Could you check a few things on this model? Use its own coordinates, in mm. Face numbers are marked on the shaded views. Give positions to 0.01 mm unless a question says otherwise; leave off trailing zeros. Loops run counter-clockwise (first coordinate to the right, second up) from the corner with the lowest first, then second, coordinate; pieces in that order, holes last. Notation, with made-up numbers: M -34.75,75.5 L -17.75,75.5 A5 ccw -17.75,82.5 Z; hole C -40,-17.75 d5. An arc over 180 degrees is marked long. Answer in a Markdown table with one row per item. Add a question column.
1. Thinking about a two-plate mould opening in Y: for the marked faces 1 and 2, which applies, released by +Y, released by -Y, zero draft, split by the parting line, or undercut?
2. If we section it at B-B on x = -14: List the corners of the cut face in (y, z) for me, then the cut area to 3 significant figures.
3. If we section it at A-A on z = 4.25: List the corners of the cut face in (x, y) for me (3 decimals).
4. I need wall thicknesses on line 1 along Y through (x, z) = (-20.5, 5.75); line 2 along Y through (x, z) = (-5.5, 5.5); line 3 along X through (y, z) = (6, 1). Which ranges of each line are inside material? Lowest first, please. Write a range as from..to.
5. I'm going to push flat-ended pins straight in: pin 1 Ø1 at (y, z) = (-6.5, 0.5) entering from -X; pin 2 Ø2 at (x, z) = (-8, 3.5) entering from +Y; pin 3 Ø1.5 at (y, z) = (30.5, 5.5) entering from -X. Where does each tip first touch, or does it pass through?
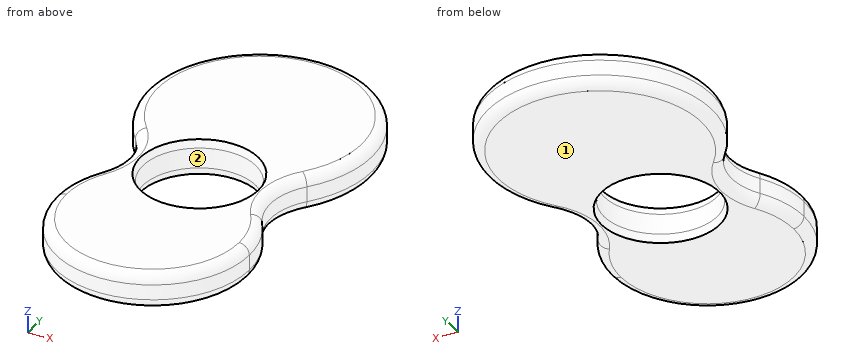
```python
from build123d import *

# Parameters (mm, degrees)
F0_R     = 11.1
F1_DEPTH = 7
F2_SIZE2 = 0.5
F2_SIZE  = 1.5
F3_R     = 2


with BuildPart() as f1:
    # F0 (on Top) → F1 (new body)
    with BuildSketch(Plane.XY):
        with BuildLine():
            ThreePointArc((-30.871365, 7.905008), (-28.023647, 0.762863), (-29.966515, -6.676558))
            ThreePointArc((-29.966515, -6.676558), (-32.225858, -11.607357), (-33, -16.975606))
            Line((-33, -16.975606), (5, -16.975606))
            ThreePointArc((5, -16.975606), (4.225858, -11.607357), (1.966515, -6.676558))
            ThreePointArc((1.966515, -6.676558), (0.023647, 0.762863), (2.871365, 7.905008))
            ThreePointArc((2.871365, 7.905008), (-14, 44.024394), (-30.871365, 7.905008))
        make_face()
        with Locations((-14, 0)):
            Circle(F0_R, mode=Mode.SUBTRACT)
        with BuildLine():
            Line((5, -16.975606), (-33, -16.975606))
            ThreePointArc((-33, -16.975606), (-14, -35.975606), (5, -16.975606))
        make_face()
    extrude(amount=F1_DEPTH)

    # F2
    f2_edges = [f1.edges().sort_by_distance(p)[0] for p in [
        (-25.1, 0, 7),
        (-25.1, 0, 0),
    ]]
    chamfer(f2_edges, length=F2_SIZE, length2=F2_SIZE2)

    # F3
    f3_edges = [f1.edges().sort_by_distance(p)[0] for p in [
        (-14, -35.975606, 7),
        (-14, -35.975606, 0),
    ]]
    fillet(f3_edges, radius=F3_R)


solid = f1.part
```
Results:
| question | item | result |
|---|---|---|
| 1 | face 1 | zero draft |
| 1 | face 2 | undercut |
| 2 | outline | M -35.98,2 A2 ccw -33.98,0 L -11.6,0 L -11.1,1.5 L -11.1,5.5 L -11.6,7 L -33.98,7 A2 ccw -35.98,5 Z; M 11.1,1.5 L 11.6,0 L 42.02,0 A2 ccw 44.02,2 L 44.02,5 A2 ccw 42.02,7 L 11.6,7 L 11.1,5.5 Z |
| 2 | area | 400 mm2 |
| 3 | outline | M -33,-16.976 A19 ccw 5,-16.976 A19 ccw 1.967,-6.677 A12.317 cw 2.871,7.905 A22 ccw long -30.871,7.905 A12.317 cw -29.967,-6.677 A19 ccw Z; hole C -14,0 d22.2 |
| 4 | line 1 | -34.67..-9.1, 9.1..42.89 |
| 4 | line 2 | -33.9..-7.14, 7.14..42.25 |
| 4 | line 3 | -29.25..-23.54, -4.46..1.25 |
| 5 | pin 1 | x = -29.65 |
| 5 | pin 2 | y = 43.45 |
| 5 | pin 3 | x = -34.57 |
